```python
from build123d import *

# Parameters (mm, degrees)
PAD_DEPTH            = 82
POCKET_DEPTH         = 3
POCKET001_DEPTH      = 2
POCKET002_DEPTH      = 2
SKETCH007_W          = 17.883893
SKETCH007_H          = 27.618155
POCKET003_DEPTH      = 1
SKETCH009_W          = 19.921296
SKETCH009_H          = 43.238262
POCKET004_DEPTH      = 4
BODY_PLACEMENT_ANGLE = 90


with BuildPart() as part:
    # Sketch → Pad (new body)
    with BuildSketch(Plane.XY):
        Polygon((30.506308, 10.196762), (-29.890312, 10.196762), (-29.890312, 49.718979), (0, 75.324928), (30.506308, 50.553959), align=None)
    extrude(amount=PAD_DEPTH)

    # Sketch001 (on Face7 of Pad) → Pocket (cut)
    with BuildSketch(Plane.XY.offset(82)):
        with BuildLine():
            Line((-25.5156, 10.058528), (-25.5156, 37.7992))
            add(Edge.make_bspline(
                [(-25.5156, 37.7992), (-20.1793, 45.2511), (-12.6602, 37.5736), (-12.6602, 37.5736), (-12.6602, 37.5736)],
                knots=[0, 0, 0, 0, 0.5, 1, 1, 1, 1], degree=3))
            Line((-12.6602, 37.5736), (-12.6602, 10.058528))
            Line((-12.6602, 10.058528), (-25.5156, 10.058528))
        make_face()
    extrude(amount=-POCKET_DEPTH, mode=Mode.SUBTRACT)

    # Sketch002 (on Face4 of Pocket) → Pocket001 (cut)
    with BuildSketch(Plane.XY.offset(82)):
        Polygon((0, 68.922791), (-22.583693, 49.75243), (22.297503, 49.75243), align=None)
    extrude(amount=-POCKET001_DEPTH, mode=Mode.SUBTRACT)

    # Sketch003 (on Face8 of Pocket001) → Pocket002 (cut)
    with BuildSketch(Plane.YZ.offset(30.506308)):
        Polygon((31.822407, 71.672646), (31.822407, 46.41288), (44.903366, 45.736275), (44.903366, 71.672646), align=None)
        Polygon((32.047943, 36.263863), (44.45229, 36.263863), (44.45229, 11.455163), (32.047943, 11.004096), align=None)
    extrude(amount=-POCKET002_DEPTH, mode=Mode.SUBTRACT)

    # Sketch007 (on Face9 of Pocket002) → Pocket003 (cut)
    with BuildSketch(Plane(origin=(-37.216188, 43.443166, 0), x_dir=(-0.759436, -0.650582, 0), z_dir=(-0.650582, 0.759436, 0))):
        with Locations((-37.439836, 21.282723)):
            Rectangle(SKETCH007_W, SKETCH007_H)
    extrude(amount=-POCKET003_DEPTH, mode=Mode.SUBTRACT)

    # Sketch009 (on Face3 of Pocket003) → Pocket004 (cut)
    with BuildSketch(Plane(origin=(-29.890312, 0, 0), x_dir=(0, -1, 0), z_dir=(-1, 0, 0))):
        with Locations((-37.215107, 41.792734)):
            Rectangle(SKETCH009_W, SKETCH009_H)
    extrude(amount=-POCKET004_DEPTH, mode=Mode.SUBTRACT)


with BuildPart() as part_1:
    # Body placement: moved
    add(part.part.rotate(Axis((0, 0, 0), (1, 0, 0)), BODY_PLACEMENT_ANGLE))


solid = part_1.part
```
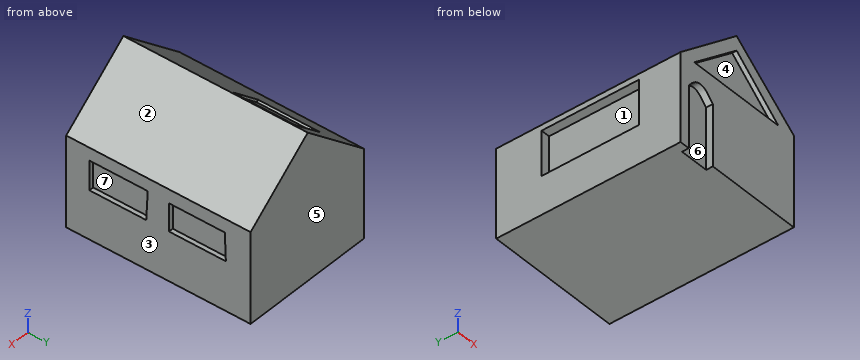
Here's how the part is built. I have some questions about the finished solid (model axes, mm). Face numbers are marked on the shaded views. A direction names the side the tool comes from. Coordinates: 2 decimals unless noted, no trailing zeros. Order: outer loops, then holes, each group sorted by start corner. A loop starts at its lowest first (then second) coordinate and runs counter-clockwise, first axis right, second up. Notation, with made-up numbers: M 44,15 L 48,15 A32 ccw 48,52 Z; hole C 25,77 d5. An arc over 180 degrees is marked long. Answer as a JSON object with one key per item and string values. Group by question number.
(1) Which directions (+Z, -Z, +X, -X, +Y, -Y) give clear straight access to the entire face, cutting with the end or side of a thin tool? Please do the marked faces 4, 5, 6 and 7.
(2) I need wall thicknesses on probe 1 along Y at (x, z) = (-17, 31.5); probe 2 along X at (y, z) = (-16, 33); probe 3 along X at (y, z) = (-49, 40.5). Which ranges of each line are inside material? Lowest first, please.
(3) If we mould it in two halves opening along Z, with no side actions, what happens to the marked faces 1, 2 and 3? For each: released by +Z, released by -Z, zero draft, split by the parting line, or undercut.
(4) For pin 1 (1.5 mm diameter, centred on x = -14, z = 32, fed in from -Y); pin 2 (6 mm diameter, centred on x = 0.5, z = 59, fed in from -Y); pin 3 (3 mm diameter, centred on x = -4.5, y = -69.5, fed in from +Z), each with a flat end and sliding along its axis, tell me the tip position at first contact or that it passes through.
(5) Suppose I cut it at B-B, the plane x = -6. Please give me the cut outline in (y, z).
(6) Suppose I cut it at A-A, the plane y = -65.5. Please give me the cut outline in (x, z), then the cut area to 3 significant figures.
(7) Suppose I cut it at D-D, the plane y = -40. Please give me the cut outline in (x, z).
(8) Suppose I cut it at C-C, the plane z = 64.5. Please give me the cut outline in (x, y).
Values found:
{
 "1": {"face 4": "-Y", "face 5": "+Z, -Z, +X, -X, +Y", "face 6": "-Z, -Y", "face 7": "+X"},
 "2": {"probe 1": "y = -79 to 0", "probe 2": "x = -29.89 to 28.51", "probe 3": "x = -25.89 to 28.51"},
 "3": {"face 1": "undercut", "face 2": "released by +Z", "face 3": "zero draft"},
 "4": {"pin 1": "stops at y = -79", "pin 2": "stops at y = -80", "pin 3": "stops at z = 72.75"},
 "5": {"outline": "M -82,10.2 L 0,10.2 L 0,70.18 L -7.47,70.18 L -7.47,68.87 L -35.09,68.87 L -35.09,70.18 L -82,70.18 L -82,63.83 L -80,63.83 L -80,49.75 L -82,49.75 Z"},
 "6": {"outline": "M -29.89,10.2 L 30.51,10.2 L 30.51,31.82 L 28.51,31.82 L 28.51,44.9 L 30.51,44.9 L 30.51,50.55 L 0,75.32 L -29.89,49.72 Z", "area": "3,150 mm^2"},
 "7": {"outline": "M -29.89,10.2 L 30.51,10.2 L 30.51,50.55 L 0,75.32 L -29.89,49.72 L -29.89,47.18 L -25.89,47.18 L -25.89,27.25 L -29.89,27.25 Z"},
 "8": {"outline": "M -12.64,-82 L -5.21,-82 L -5.21,-80 L 5.14,-80 L 5.14,-82 L 13.33,-82 L 13.33,0 L -12.64,0 L -12.64,-7.47 L -11.1,-7.47 L -11.1,-35.09 L -12.64,-35.09 Z"}
}
